Build history of the part. All positions in model axes, mm. Coordinates: 2 decimals unless noted, no trailing zeros. Order: outer loops, then holes, each group sorted by start corner. A loop starts at its lowest first (then second) coordinate and runs counter-clockwise, first axis right, second up. Notation, with made-up numbers: (65, 54.25) - (121, 54.25) arc R17 cw to (121, 62.25) - close; hole circle Ø2 at (50, 62). An arc over 180 degrees is marked (long way). Write each question's results on one line, items separated by ' | '.
from build123d import *

# Parameters (mm, degrees)
SKETCH1_R           = 76.2
SKETCH1_R_2         = 74.549
BOSS_EXTRUDE1_DEPTH = 254
WRAP2_SECTION_W     = 3.302
WRAP2_SECTION_H     = 101.6
WRAP2_ANGLE         = 76.394372684


with BuildPart() as part:
    # Sketch1 → Boss-Extrude1 (new body)
    with BuildSketch(Plane(origin=(0, 0, 0), x_dir=(1, 0, 0), z_dir=(0, 1, 0))):
        with Locations(Location((0, 0, 0), (0, 0, 270))):
            Circle(SKETCH1_R)
        with Locations(Location((0, 0, 0), (0, 0, 270))):
            Circle(SKETCH1_R_2, mode=Mode.SUBTRACT)
    extrude(amount=BOSS_EXTRUDE1_DEPTH)

    # Wrap2 section (on wrap section) → Wrap2 (revolve, cut)
    with BuildSketch(Plane(origin=(0, 0, 0), x_dir=(0.6183698030697371, 0, 0.7858872607769479), z_dir=(0.7858872607769479, 0, -0.6183698030697371))):
        with Locations((74.549, -127)):
            Rectangle(WRAP2_SECTION_W, WRAP2_SECTION_H)
    revolve(axis=Axis((0, 0, 0), (0, -1, 0)), revolution_arc=WRAP2_ANGLE, mode=Mode.SUBTRACT)


solid = part.part
1. Two-plate mould, pull along Y, no slides. Class faces 1 (the face through (-56, 0, 50)), 2 (the face through (1, 177.8, 75)), 3 (the face through (-56, 254, 50)): +Y half, -Y half, draft (parallel to the pull), parting line (faces both ways), or undercut.
Solved:
face 1: -Y half | face 2: undercut | face 3: +Y half
2. Band-saw the part on D-D on y = 173. Give the cut face in (x, z).
Solved:
outline: (-47.12, 59.88) arc R76.2 ccw (long way) to (47.12, 59.88) - (46.1, 58.59) arc R74.55 cw (long way) to (-46.1, 58.59) - close
3. Band-saw the part on B-B on z = 0. Give the cut face in (x, y).
Solved:
outline: (-76.2, 0) - (-74.55, 0) - (-74.55, 254) - (-76.2, 254) - close; (74.55, 0) - (76.2, 0) - (76.2, 254) - (74.55, 254) - close
4. Band-saw the part on A-A on x = 0. Give the cut face in (y, z).
Solved:
outline: (0, -76.2) - (254, -76.2) - (254, -74.55) - (0, -74.55) - close; (0, 74.55) - (76.2, 74.55) - (76.2, 76.2) - (0, 76.2) - close; (177.8, 74.55) - (254, 74.55) - (254, 76.2) - (177.8, 76.2) - close
5. Band-saw the part on C-C on x = 51. Give the cut face in (y, z).
Solved:
outline: (0, -56.62) - (254, -56.62) - (254, -54.37) - (0, -54.37) - close; (0, 54.37) - (254, 54.37) - (254, 56.62) - (0, 56.62) - close
6. Probe line 1 (X direction, y = 77, z = 0); line 2 (Z direction, x = 2.5, y = 191.5); line 3 (X direction, y = 209, z = -64.5). List the from-to ranges inside material, lowest first.
Solved:
line 1: x = -76.2 to -74.55, 74.55 to 76.2 | line 2: z = -76.16 to -74.51, 74.51 to 76.16 | line 3: x = -40.57 to -37.38, 37.38 to 40.57
7. Drop flat-ended pins along their axis: pin 1 Ø10 at (x, y) = (-37, 122) entering from +Z; pin 2 Ø6 at (x, y) = (4, 160) entering from +Z; pin 3 Ø3 at (x, y) = (38.5, 199) entering from -Z. Give the stop position or say it passes through.
Solved:
pin 1: stops at z = -61.59 | pin 2: stops at z = -74.22 | pin 3: stops at z = -66.61
